The listing builds one solid part. Answer for the finished solid, in the listing's coordinates (mm). A direction names the side the tool comes from. Give positions to 0.01 mm unless a question says otherwise; leave off trailing zeros. Order: outer loops, then holes, each group sorted by start corner. A loop starts at its lowest first (then second) coordinate and runs counter-clockwise, first axis right, second up.
Autodesk Inventor part; units mm, degrees
ref_plane "YZ Plane" through (0, 0, 0) normal (1, 0, 0) x (0, 1, 0)
ref_plane "XZ Plane" through (0, 0, 0) normal (0, 1, 0) x (-1, 0, 0)
ref_plane "XY Plane" through (0, 0, 0) normal (0, 0, 1) x (1, 0, 0)
sketch "Sketch1" plane through (0, 0, 0) normal (0, 0, 1) x (1, 0, 0)
  line L0 (0, 0) -> (60, 0)
  line L1 (60, 0) -> (60, 8)
  line L2 (60, 8) -> (0, 8)
  line L3 (0, 8) -> (0, 0)
  dimension "d0" = 60
  dimension "d3" = 8
extrude "Extrusion1" add sketch "Sketch1" along normal blind 6
sketch "Sketch2" plane through (0, 0, 6) normal (0, 0, 1) x (1, 0, 0)
  line L0 (0, 0) -> (60, 0)
  line L1 (2, 1.5) -> (58, 1.5)
  line L2 (60, 0) -> (60, 8)
  line L3 (2, 1.5) -> (2, 8)
  line L4 (60, 8) -> (0, 8)
  line L5 (58, 1.5) -> (58, 8)
  line L6 (58, 8) -> (2, 8)
  line L7 (0, 4.6) -> (60, 4.6) construction
  dimension "d5" = 1.5
  dimension "d6" = 56
  dimension "d7" = 2
  dimension "d12" = 4.6
extrude "Extrusion2" cut sketch "Sketch2" against normal blind 20
sketch "Sketch3" plane through (0, 0, 6) normal (0, 0, 1) x (1, 0, 0)
  line L0 (0, 8) -> (0, 0) construction
  line L1 (0, 4.6) -> (60, 4.6) construction
  line L2 (60, 0) -> (60, 8) construction
  line L3 (0, 0) -> (60, 0) construction
  line L4 (2, 1.5) -> (2, 8) construction
  arc A0 (2, 4.6) -> (2, 5.6) centre (2, 5.1) ccw
  line L5 (2, 5.6) -> (2, 4.6)
  line L6 (58, 1.5) -> (58, 8)
  arc A1 (58, 5.6) -> (58, 4.6) centre (58, 5.1) ccw
  line L7 (58, 5.6) -> (58, 4.6)
  dimension "d13" = 4.6
  dimension "d17" = 1
  dimension "d18" = 5.1
  dimension "d19" = 1
  dimension "d20" = 5.1
extrude "Extrusion3" add sketch "Sketch3" against normal blind 6
properties part number "Houderpi"
1) Find section A-A (y = 5.1). Write down the section's boundary in (x, z).
Geometry says:
outline: (0, 0) - (2.5, 0) - (2.5, 6) - (0, 6) - close; (57.5, 0) - (60, 0) - (60, 6) - (57.5, 6) - close
2) For a pull along X with two mould halves and no side action, classify faces 4 (the flat face through (0, 4, 3)), 5 (the flat face through (60, 4, 3)), 6 (the flat face through (1, 8, 3)), 7 (the flat face through (2, 7, 3)) as +X half, -X half, draft (parallel to the pull), parting line (faces both ways), or undercut.
Geometry says:
face 4: -X half
face 5: +X half
face 6: draft
face 7: undercut
3) Find section B-B (z = 1.9). Write down the section's boundary in (x, y), then the cut area to 3 significant figures.
Geometry says:
outline: (0, 0) - (60, 0) - (60, 8) - (58, 8) - (58, 5.6) arc R0.5 ccw to (58, 4.6) - (58, 1.5) - (2, 1.5) - (2, 4.6) arc R0.5 ccw to (2, 5.6) - (2, 8) - (0, 8) - close
area: 117 mm2
4) Straight lines are drawn through the part: probe 1 along X at (y, z) = (4, 2.7); probe 2 along Y at (x, z) = (50, 4.15); probe 3 along X at (y, z) = (4.75, 5.3). For each, find the intervals that lie inside material, in ascending order.
Geometry says:
probe 1: x = 0 to 2, 58 to 60
probe 2: y = 0 to 1.5
probe 3: x = 0 to 2.36, 57.64 to 60
5) Find section C-C (x = 26.5). Write down the section's boundary in (y, z), then the cut area to 3 significant figures.
Geometry says:
outline: (0, 0) - (1.5, 0) - (1.5, 6) - (0, 6) - close
area: 9.00 mm2
6) A tool of negligible diameter and unlimited length cuts with its end or side. For faces 1 (the flat face through (59, 8, 3)), 2 (the flat face through (2, 3, 3)), 3 (the flat face through (58, 7, 3)), from which of +Z, -Z, +X, -X, +Y, -Y can it reach the whole face along a straight path? Write none if from no direction.
Geometry says:
face 1: +Z, -Z, +X, -X, +Y
face 2: +Z, -Z
face 3: +Z, -Z, +Y
